Design review of the part built by this model. Coordinates are the model's own, in mm. Coordinates: 2 decimals unless noted, no trailing zeros. Write each loop counter-clockwise with the first axis right and the second up, starting at its lowest first coordinate (ties: lowest second). Pieces come first, ordered by that corner, then holes. Notation, with made-up numbers: (24.5, 71) -> (83.5, 71) arc R25 cw to (83.5, 99) -> close; hole circle Ø7 at (28, -6). An arc over 180 degrees is marked (long way). Answer in a Markdown table with one row per item. Add a question column.
Item 1: Take a section at A-A, the plane y = 1.2. Write out the cut boundary in (x, z).
Item 2: To check wall thickness, follow line 1 (X direction, y = 3.3, z = 0); line 2 (X direction, y = 0.5, z = -9.25); line 3 (Z direction, x = -5.5, y = 3.6). State the ranges of each line that lie inside material, in increasing order.
Item 3: Draft analysis for pull direction X (two halves, no side actions). For faces 1 (the face through (13.05, 2.47, -7.4)), 2 (the face through (-2.222, 2.465, 10.006)), 3 (the face through (10, 0, 3)), state which applies: released by +X, released by -X, zero draft, split by the parting line, or undercut.
Item 4: Clearance check with a flat-ended pin moving along its axis: P1, Ø2, axis at y = 1.5, z = -6.5, coming from the -X side. State where the tip first meets the part, or that it passes through.
from build123d import *

# Parameters (mm, degrees)
SKETCH_1_R          = 10.25
EXTRUDE_1_DEPTH     = 5
SKETCH_2_OUTSIDE_W  = 97.84
SKETCH_2_OUTSIDE_H  = 93.198
SKETCH_2_OUTSIDE_R  = 15
CUT_EXTRUDE_1_DEPTH = 6
CUT_EXTRUDE_1_TAPER = 77
SKETCH_3_OUTSIDE_W  = 97.84
SKETCH_3_OUTSIDE_H  = 93.198
SKETCH_3_OUTSIDE_R  = 15
CUT_EXTRUDE_2_DEPTH = 6
CUT_EXTRUDE_2_TAPER = 77


with BuildPart() as part:
    # Эскиз1 → Бобышка-Вытянуть1 (new body)
    with BuildSketch(Plane(origin=(0, 0, 0), x_dir=(1, 0, 0), z_dir=(0, 1, 0))):
        Polygon((17.320508076, 0), (8.660254038, 15), (-8.660254038, 15), (-17.320508076, 0), (-8.660254038, -15), (8.660254038, -15), align=None)
        Circle(SKETCH_1_R, mode=Mode.SUBTRACT)
    extrude(amount=EXTRUDE_1_DEPTH)

    # Эскиз2 outside → Вырез-Вытянуть1 (cut, through all)
    with BuildSketch(Plane(origin=(0, 5, 0), x_dir=(1, 0, 0), z_dir=(0, 1, 0))):
        Rectangle(SKETCH_2_OUTSIDE_W, SKETCH_2_OUTSIDE_H)
        Circle(SKETCH_2_OUTSIDE_R, mode=Mode.SUBTRACT)
    extrude(amount=-CUT_EXTRUDE_1_DEPTH, taper=CUT_EXTRUDE_1_TAPER, mode=Mode.SUBTRACT)

    # Эскиз3 outside → Вырез-Вытянуть2 (cut, through all)
    with BuildSketch(Plane.XZ):
        Rectangle(SKETCH_3_OUTSIDE_W, SKETCH_3_OUTSIDE_H)
        Circle(SKETCH_3_OUTSIDE_R, mode=Mode.SUBTRACT)
    extrude(amount=-CUT_EXTRUDE_2_DEPTH, taper=CUT_EXTRUDE_2_TAPER, mode=Mode.SUBTRACT)


solid = part.part
Answers:
| question | item | result |
|---|---|---|
| 1 | outline | (-17.32, 0) -> (-8.66, -15) -> (8.66, -15) -> (17.32, 0) -> (8.66, 15) -> (-8.66, 15) -> close; hole circle Ø20.5 at (0, 0) |
| 2 | line 1 | x = -17.32 to -10.25, 10.25 to 17.32 |
| 2 | line 2 | x = -11.98 to -4.42, 4.42 to 11.98 |
| 2 | line 3 | z = -15 to -8.65, 8.65 to 15 |
| 3 | face 1 | released by +X |
| 3 | face 2 | undercut |
| 3 | face 3 | zero draft |
| 4 | P1 | stops at x = -14.15 |
